```python
from build123d import *

# Parameters (mm, degrees)
SKETCH_1_W               = 30
SKETCH_1_H               = 30
EXTRUDE_1_DEPTH          = 5.8
EXTRUDE_2_DEPTH          = 25.2
SKETCH_3_W               = 18
SKETCH_3_H               = 18
CUT_EXTRUDE_1_DEPTH      = 1
EXTRUDE_4_DEPTH          = 25
PATTERN_CIRCULAR_1_COUNT = 2
PATTERN_CIRCULAR_1_ANGLE = 90
HOLE_WIZARD_M6_1_D       = 5
HOLE_WIZARD_M6_2_D       = 5
HOLE_WIZARD_M6_3_D       = 5
FILLET_1_R               = 2.5


with BuildPart() as part:
    # 草图1 → 凸台-拉伸1 (new body)
    with BuildSketch(Plane(origin=(0, 0, 0), x_dir=(1, 0, 0), z_dir=(0, 1, 0))):
        Rectangle(SKETCH_1_W, SKETCH_1_H)
    extrude(amount=EXTRUDE_1_DEPTH)

    # 草图2 → 凸台-拉伸2 (add)
    with BuildSketch(Plane(origin=(0, 0, 0), x_dir=(-1, 0, 0), z_dir=(0, -1, 0))):
        Polygon((4, -15), (4, -13), (8, -13), (8, -11.5), (5.5, -9), (-5.5, -9), (-8, -11.5), (-8, -13), (-4, -13), (-4, -15), align=None)
        Polygon((15, 4), (13, 4), (13, 8), (11.5, 8), (9, 5.5), (9, -5.5), (11.5, -8), (13, -8), (13, -4), (15, -4), align=None)
    extrude(amount=EXTRUDE_2_DEPTH)

    # 草图3 → 切除-拉伸1 (cut)
    with BuildSketch(Plane.XZ):
        Rectangle(SKETCH_3_W, SKETCH_3_H)
    extrude(amount=-CUT_EXTRUDE_1_DEPTH, mode=Mode.SUBTRACT)

    # 草图5 → 凸台-拉伸4 (add)
    with BuildSketch(Plane(origin=(0, 0, -15), x_dir=(-1, 0, 0), z_dir=(0, 0, -1))):
        Polygon((-5.5, 0), (5.5, 0), (8, 2.5), (8, 3.8), (4, 3.8), (4, 5.8), (-4, 5.8), (-4, 3.8), (-8, 3.8), (-8, 2.5), align=None)
    extrude_4 = extrude(amount=EXTRUDE_4_DEPTH)

    # 阵列(圆周)1: 凸台-拉伸4 ×2 about axis
    pattern_circular_1_axis = Axis((0, 0, 0), (0, -1, 0))
    for i in range(1, PATTERN_CIRCULAR_1_COUNT):
        add(extrude_4.rotate(pattern_circular_1_axis, i * PATTERN_CIRCULAR_1_ANGLE / (PATTERN_CIRCULAR_1_COUNT - 1)))

    # M6 螺纹孔1 (through all)
    with Locations(Plane(origin=(0, 0, 0), x_dir=(-1, 0, 0), z_dir=(0, -1, 0))):
        with Locations((-30, 0), (0, 30)):
            Hole(HOLE_WIZARD_M6_1_D / 2)

    # M6 螺纹孔2 (through all)
    with Locations(Plane.ZY.offset(15)):
        with Locations((0, -15.2)):
            Hole(HOLE_WIZARD_M6_2_D / 2)

    # M6 螺纹孔3 (through all)
    with Locations(Plane.XY.offset(15)):
        with Locations((0, -15.2)):
            Hole(HOLE_WIZARD_M6_3_D / 2)

    # 圆角1
    fillet_1_edges = [part.edges().sort_by_distance(p)[0] for p in [
        (15, 2.9, 15),
        (-15, 2.9, 15),
        (-15, 2.9, -15),
        (15, 2.9, -15),
    ]]
    fillet(fillet_1_edges, radius=FILLET_1_R)


solid = part.part
```
Here's how the part is built. I have some questions about the finished solid (model axes, mm). A direction names the side the tool comes from. Coordinates: 2 decimals unless noted, no trailing zeros. Loops run counter-clockwise (first coordinate to the right, second up) from the corner with the lowest first, then second, coordinate; pieces in that order, holes last. Notation, with made-up numbers: (58, 32) - (104, 32) arc R16 cw to (104, 51) - close; hole circle Ø7 at (-40, 16). An arc over 180 degrees is marked (long way). Return JSON: item names as keys, results as strings. Group by question number.
Item 1: I need wall thicknesses on line 1 (Z direction, x = 0, y = 3.3); line 2 (Y direction, x = -11, z = 0); line 3 (X direction, y = 3.65, z = -30). Which ranges of each line are inside material? Lowest first, please. Write a range as from..to.
Item 2: If we section it at C-C on y = -14.5: Write out the boundary of the cut face in (x, z), and give its area (3 significant figures).
Item 3: On a 3-axis mill with a long thin cutter (end or side, diameter ignored), from which of +Z, -Z, +X, -X, +Y, -Y can I reach the whole of each face in a straight line? I mean faces 1 (the face through (27.3, 1.2, -6.7)), 2 (the face through (-12, -12, -8)), 3 (the face through (4, 5, -27)), 4 (the face through (-8, -12, 12)), 5 (the face through (-4, -12, 14)). Say none if no direction works.
Item 4: If we section it at D-D on x = 0: Write out the boundary of the cut face in (y, z).
Item 5: If we section it at A-A on x = 30: Write out the boundary of the cut face in (y, z), and give its area (4 significant figures).
Item 6: We'd pull the mould along Y, two halves only. Please class faces 6 (the face through (0, 5.8, -1)), 7 (the face through (6.7, -12.4, 10.2)), 8 (the face through (-11.96, -12.72, 0.33)): +Y half, -Y half, draft (parallel to the pull), parting line (faces both ways), or undercut.
Item 7: If we section it at B-B on z = 0: Write out the boundary of the cut face in (x, y), and give its area (3 significant figures).
Item 8: Will these pins go through, and if not, where does the flat tip stop? P1, Ø4, axis at y = -15.2, z = 0, coming from the +X side; P2, Ø0.6, axis at y = 5, z = -31.5, coming from the +X side; P3, Ø2, axis at y = -17.5, z = -6.5, coming from the -X side; P4, Ø3, axis at x = 31.5, y = 2, coming from the +Z side.
Calculated:
{
 "1": {"line 1": "z = -40..-32.5, -27.5..15", "line 2": "y = -25.2..-17.7, -12.7..5.8", "line 3": "x = -8..-2.5, 2.5..8"},
 "2": {"outline": "(-15, -4) - (-13, -4) - (-13, -8) - (-11.5, -8) - (-9, -5.5) - (-9, -2.4) - (-15, -2.4) - close; (-15, 2.4) - (-9, 2.4) - (-9, 5.5) - (-11.5, 8) - (-13, 8) - (-13, 4) - (-15, 4) - close; (-8, 11.5) - (-5.5, 9) - (-2.4, 9) - (-2.4, 15) - (-4, 15) - (-4, 13) - (-8, 13) - close; (2.4, 9) - (5.5, 9) - (8, 11.5) - (8, 13) - (4, 13) - (4, 15) - (2.4, 15) - close", "area": "89.9 mm^2"},
 "3": {"face 1": "-Z, +X, -Y", "face 2": "-Z, +X, -X, -Y", "face 3": "-Z, +X, +Y", "face 4": "+Z, -Z, -X, -Y", "face 5": "+Z, -X, -Y"},
 "4": {"outline": "(-25.2, 9) - (-17.7, 9) - (-17.7, 15) - (-25.2, 15) - close; (-12.7, 9) - (1, 9) - (1, -9) - (0, -9) - (0, -27.5) - (5.8, -27.5) - (5.8, 15) - (-12.7, 15) - close; (0, -40) - (5.8, -40) - (5.8, -32.5) - (0, -32.5) - close"},
 "5": {"outline": "(0, -5.5) - (2.5, -8) - (3.8, -8) - (3.8, -4) - (5.8, -4) - (5.8, -2.5) - (0, -2.5) - close; (0, 2.5) - (5.8, 2.5) - (5.8, 4) - (3.8, 4) - (3.8, 8) - (2.5, 8) - (0, 5.5) - close", "area": "41.55 mm^2"},
 "6": {"face 6": "+Y half", "face 7": "draft", "face 8": "undercut"},
 "7": {"outline": "(-15, -25.2) - (-9, -25.2) - (-9, -17.7) - (-15, -17.7) - close; (-15, -12.7) - (-9, -12.7) - (-9, 1) - (9, 1) - (9, 0) - (27.5, 0) - (27.5, 5.8) - (-15, 5.8) - close; (32.5, 0) - (40, 0) - (40, 5.8) - (32.5, 5.8) - close", "area": "393 mm^2"},
 "8": {"P1": "passes through", "P2": "stops at x = 4", "P3": "stops at x = -13", "P4": "stops at z = 8"}
}
